from build123d import *
from OCP.BRepAlgoAPI import BRepAlgoAPI_Cut
from OCP.TopTools import TopTools_ListOfShape

# Parameters (mm, degrees)
SKETCH1_R           = 40
SKETCH1_R_2         = 2.5
SKETCH1_W           = 14
SKETCH1_H           = 14
BOSS_EXTRUDE1_DEPTH = 5
BOSS_EXTRUDE2_DEPTH = 5
FILLET1_R           = 5
SKETCH3_W           = 4
SKETCH3_H           = 1
CUT_EXTRUDE1_DEPTH  = 3.5


with BuildPart() as part:
    # Sketch1 → Boss-Extrude1 (new body)
    with BuildSketch(Plane(origin=(0, 0, 0), x_dir=(1, 0, 0), z_dir=(0, 1, 0))):
        with Locations(Location((0, 0, 0), (0, 0, 270))):
            Circle(SKETCH1_R)
        with Locations(Location((-19.05, 25, 0), (0, 0, 270))):
            Circle(SKETCH1_R_2, mode=Mode.SUBTRACT)
        with Locations(Location((19.05, 25, 0), (0, 0, 270))):
            Circle(SKETCH1_R_2, mode=Mode.SUBTRACT)
        with Locations(Location((19.05, -25, 0), (0, 0, 270))):
            Circle(SKETCH1_R_2, mode=Mode.SUBTRACT)
        with Locations(Location((-19.05, -25, 0), (0, 0, 270))):
            Circle(SKETCH1_R_2, mode=Mode.SUBTRACT)
        with Locations((0, 19.05)):
            Rectangle(SKETCH1_W, SKETCH1_H, mode=Mode.SUBTRACT)
        Rectangle(SKETCH1_W, SKETCH1_H, mode=Mode.SUBTRACT)
        with Locations((0, -19.05)):
            Rectangle(SKETCH1_W, SKETCH1_H, mode=Mode.SUBTRACT)
        with Locations((-19.05, 9.525)):
            Rectangle(SKETCH1_W, SKETCH1_H, mode=Mode.SUBTRACT)
        with Locations((19.05, 9.525)):
            Rectangle(SKETCH1_W, SKETCH1_H, mode=Mode.SUBTRACT)
        with Locations((-19.04999963, -9.524995038)):
            Rectangle(SKETCH1_W, SKETCH1_H, mode=Mode.SUBTRACT)
        with Locations((19.05000037, -9.524995038)):
            Rectangle(SKETCH1_W, SKETCH1_H, mode=Mode.SUBTRACT)
    extrude(amount=BOSS_EXTRUDE1_DEPTH)

    # Sketch2 → Boss-Extrude2 (add)
    with BuildSketch(Plane(origin=(0, 5, 0), x_dir=(1, 0, 0), z_dir=(0, 1, 0))):
        with BuildLine():
            Line((-39.921798557, 2.5), (-29.05, 2.5))
            Line((-29.05, 2.5), (-29.05, -2.5))
            Line((-29.05, -2.5), (-39.921798557, -2.5))
            ThreePointArc((-39.921798557, -2.5), (-40, 0), (-39.921798557, 2.5))
        make_face()
        with BuildLine():
            Line((29.05, 2.5), (29.05, -2.5))
            Line((29.05, -2.5), (39.921798557, -2.5))
            ThreePointArc((39.921798557, -2.5), (40, 0), (39.921798557, 2.5))
            Line((39.921798557, 2.5), (29.05, 2.5))
        make_face()
    extrude(amount=BOSS_EXTRUDE2_DEPTH)

    # Fillet1
    fillet1_edges = [part.edges().sort_by_distance(p)[0] for p in [
        (40, 10, 0),
        (-40, 10, 0),
    ]]
    fillet(fillet1_edges, radius=FILLET1_R - 0.0001)  # a hair under: the kernel refuses the full size


with BuildPart() as cut_extrude1_tool:
    # Sketch3 → Cut-Extrude1 (new body)
    with BuildSketch(Plane.XZ):
        with Locations((0, 26.55)):
            Rectangle(SKETCH3_W, SKETCH3_H)
        with Locations((0, 11.55)):
            Rectangle(SKETCH3_W, SKETCH3_H)
        with Locations((0, 7.5)):
            Rectangle(SKETCH3_W, SKETCH3_H)
        with Locations((0, -7.5)):
            Rectangle(SKETCH3_W, SKETCH3_H)
        with Locations((0, -11.55)):
            Rectangle(SKETCH3_W, SKETCH3_H)
        with Locations((0, -26.55)):
            Rectangle(SKETCH3_W, SKETCH3_H)
        with Locations((-19.04999963, 17.024995038)):
            Rectangle(SKETCH3_W, SKETCH3_H)
        with Locations((-19.04999963, 2.024995038)):
            Rectangle(SKETCH3_W, SKETCH3_H)
        with Locations((19.05000037, 2.024995038)):
            Rectangle(SKETCH3_W, SKETCH3_H)
        with Locations((19.05000037, 17.024995038)):
            Rectangle(SKETCH3_W, SKETCH3_H)
        with Locations((19.05000037, -17.025004962)):
            Rectangle(SKETCH3_W, SKETCH3_H)
        with Locations((19.05000037, -2.025004962)):
            Rectangle(SKETCH3_W, SKETCH3_H)
        with Locations((-19.04999963, -17.025004962)):
            Rectangle(SKETCH3_W, SKETCH3_H)
        with Locations((-19.04999963, -2.025004962)):
            Rectangle(SKETCH3_W, SKETCH3_H)
    extrude(amount=-CUT_EXTRUDE1_DEPTH)


with BuildPart() as part_1:
    add(part.part)

    # Cut-Extrude1: cut by cut_extrude1_tool, with a tolerance
    cut_extrude1_stock = TopTools_ListOfShape()
    cut_extrude1_stock.Append(part_1.part.wrapped)
    cut_extrude1_tools = TopTools_ListOfShape()
    cut_extrude1_tools.Append(cut_extrude1_tool.part.wrapped)
    cut_extrude1_cut = BRepAlgoAPI_Cut()
    cut_extrude1_cut.SetArguments(cut_extrude1_stock)
    cut_extrude1_cut.SetTools(cut_extrude1_tools)
    cut_extrude1_cut.SetFuzzyValue(0.00001)
    cut_extrude1_cut.Build()
    add(Compound.cast(cut_extrude1_cut.Shape()).solids(), mode=Mode.REPLACE)


solid = part_1.part
For this review, take the finished solid that the model builds, in its own axes (mm). A direction names the side the tool comes from. Round coordinates to 2 decimals unless told otherwise and drop trailing zeros. Write each loop counter-clockwise with the first axis right and the second up, starting at its lowest first coordinate (ties: lowest second). Pieces come first, ordered by that corner, then holes. Notation, with made-up numbers: M 37.5,59 L 87.5,59 A12 cw 87.5,69 Z; hole C 48.5,71.25 d1. An arc over 180 degrees is marked long. Write item = value, one per line. Start each with the question number.
(1) We need section B-B (x = 0). Give the boundary of the cut face in (y, z).
(2) For line 1 along X through (y, z) = (2.8, -25); line 2 along Z through (x, y) = (-4, 0.75); line 3 along X through (y, z) = (1.25, -24), list the stretches that pass through material, from the lowest coordinate up.
(3) We need section C-C (z = -23.5). Give the boundary of the cut face in (x, y), then the cut area to 3 significant figures.
(4) Clearance check with flat-ended pins moving along their axes: pin 1 Ø0.8 at (y, z) = (2.5, -2) entering from -X; pin 2 Ø4 at (y, z) = (2, -17) entering from -X; pin 3 Ø1.5 at (y, z) = (3.5, 28.5) entering from +X. State where each tip first meets the part, or that it passes through.
(5) We need section D-D (x = -19.05). Give the boundary of the cut face in (y, z) (3 decimals), then the cut area to 3 significant figures.
(6) We need section A-A (z = 0). Give the boundary of the cut face in (x, y).
(7) For faces 1 (the face through (29.05, 7, 0)), 2 (the face through (19, 2, 17.525)), 3 (the face through (35, 7, -2.5)), 4 (the face through (-19, 4, -2.525)), list the 3-axis set-ups (+Z, -Z, +X, -X, +Y, -Y) from which the entire face can be reached by the end or side of a thin tool; tool diameter is ignored.
Results found:
q1.outline = M 0,-40 L 5,-40 L 5,-26.05 L 3.5,-26.05 L 3.5,-27.05 L 0,-27.05 Z; M 0,-11.05 L 3.5,-11.05 L 3.5,-12.05 L 5,-12.05 L 5,-7 L 3.5,-7 L 3.5,-8 L 0,-8 Z; M 0,8 L 3.5,8 L 3.5,7 L 5,7 L 5,12.05 L 3.5,12.05 L 3.5,11.05 L 0,11.05 Z; M 0,27.05 L 3.5,27.05 L 3.5,26.05 L 5,26.05 L 5,40 L 0,40 Z
q2.line_1 = -31.22 to -21.55, -16.55 to -7, 7 to 16.55, 21.55 to 31.22
q2.line_2 = -39.8 to -26.05, -12.05 to -7, 7 to 12.05, 26.05 to 39.8
q2.line_3 = -32 to -21.34, -16.76 to -7, 7 to 16.76, 21.34 to 32
q3.outline = M -32.37,0 L -21.05,0 L -21.05,5 L -32.37,5 Z; M -17.05,0 L -7,0 L -7,5 L -17.05,5 Z; M 7,0 L 17.05,0 L 17.05,5 L 7,5 Z; M 21.05,0 L 32.37,0 L 32.37,5 L 21.05,5 Z
q3.area = 214 mm²
q4.pin_1 = -39.97
q4.pin_2 = -37.08
q4.pin_3 = 28.81
q5.outline = M 0,-35.172 L 5,-35.172 L 5,-27.5 L 0,-27.5 Z; M 0,-22.5 L 5,-22.5 L 5,-16.525 L 3.5,-16.525 L 3.5,-17.525 L 0,-17.525 Z; M 0,-1.525 L 3.5,-1.525 L 3.5,-2.525 L 5,-2.525 L 5,2.525 L 3.5,2.525 L 3.5,1.525 L 0,1.525 Z; M 0,17.525 L 3.5,17.525 L 3.5,16.525 L 5,16.525 L 5,22.5 L 0,22.5 Z; M 0,27.5 L 5,27.5 L 5,35.172 L 0,35.172 Z
q5.area = 148 mm²
q6.outline = M -40,0 L -7,0 L -7,5 L -29.05,5 L -29.05,10 L -35,10 A5 ccw -40,5 Z; M 7,0 L 40,0 L 40,5 A5 ccw 35,10 L 29.05,10 L 29.05,5 L 7,5 Z
q7.face_1 = +Z, -Z, +Y
q7.face_2 = -Y
q7.face_3 = -Z, +X, -X, +Y
q7.face_4 = +Y, -Y
